Autodesk Inventor part; units mm, degrees
ref_plane "YZ Plane" through (0, 0, 0) normal (1, 0, 0) x (0, 1, 0)
ref_plane "XZ Plane" through (0, 0, 0) normal (0, 1, 0) x (-1, 0, 0)
ref_plane "XY Plane" through (0, 0, 0) normal (0, 0, 1) x (1, 0, 0)
sketch "Sketch1" plane through (0, 0, 0) normal (0, 1, 0) x (-1, 0, 0)
  line L0 (0, 0) -> (76.2, 0)
  line L1 (76.2, 0) -> (76.2, 25.4)
  line L2 (76.2, 25.4) -> (0, 25.4)
  line L3 (0, 25.4) -> (0, 0)
  line L4 (7.9375, 12.7) -> (68.2625, 12.7) construction
  circle A0 centre (7.9375, 12.7) radius 3.302
  circle A1 centre (68.2625, 12.7) radius 3.302
  line L5 (38.1, 25.4) -> (38.1, 0) construction
  point P0 (38.1, 12.7)
  dimension "d0" = 76.2
  dimension "d1" = 6.604
  dimension "d2" = 60.325
  dimension "d3" = 25.4
extrude "Extrusion1" add sketch "Sketch1" along normal blind 3.175
fillet "Fillet1" radius 3.175 4 edges at (0, 1.5875, 25.4) (0, 1.5875, 0) (-76.2, 1.5875, 25.4) (-76.2, 1.5875, 0)
properties part number "Wheel Mount Support Plate - drive wheel" material "Aluminum 6061"
Can you work these out from the model? Positions are in its coordinate system, mm. Give positions to 0.01 mm unless a question says otherwise; leave off trailing zeros. Loops run counter-clockwise (first coordinate to the right, second up) from the corner with the lowest first, then second, coordinate; pieces in that order, holes last. Notation, with made-up numbers: M 31.5,67 L 61.5,67 A15 ccw 61.5,73 Z; hole C 7.5,10 d1. An arc over 180 degrees is marked long. Use one line per item in the form item = value. Start each with the question number.
(1) I want a section at A-A, the plane z = 12.7. Write out the boundary of the cut face in (x, y) (1 decimal).
(2) I want a section at B-B, the plane y = 1.35. State how many separate pieces and enclosed holes the cut face has, and give its area (3 significant figures).
(3) Thinking about a two-plate mould opening in Z: for faces 1 (the flat face through (-38, 3.175, 13)), 2 (the cylindrical face through (-0.91, 1.61, 0.95)), 3 (the cylindrical face through (-69.786, 1.565, 15.629)), 4 (the cylindrical face through (-75.29, 1.61, 24.45)), which applies, released by +Z, released by -Z, zero draft, split by the parting line, or undercut?
(4) Please list where these lines run through material, in increasing order: line 1 (Z direction, x = -7, y = 2.6); line 2 (Z direction, x = -6.5, y = 1.05); line 3 (X direction, y = 2.35, z = 3).
(5) I'm going to push a flat-ended pin straight in: P1, Ø2, axis at x = -65, z = 22, coming from the -Y side. Where does the tip first touch, or does it pass through?
Worked out:
q1.outline = M -76.2,0 L -71.6,0 L -71.6,3.2 L -76.2,3.2 Z; M -65,0 L -11.2,0 L -11.2,3.2 L -65,3.2 Z; M -4.6,0 L 0,0 L 0,3.2 L -4.6,3.2 Z
q2.separate_pieces = 1
q2.enclosed_holes = 2
q2.area = 1,860 mm²
q3.face_1 = zero draft
q3.face_2 = released by -Z
q3.face_3 = undercut
q3.face_4 = released by +Z
q4.line_1 = 0 to 9.53, 15.87 to 25.4
q4.line_2 = 0 to 9.73, 15.67 to 25.4
q4.line_3 = -76.2 to 0
q5.P1 = 0
